Can you work these out from the model? Positions are in its coordinate system, mm. Coordinates: 2 decimals unless noted, no trailing zeros. Order: outer loops, then holes, each group sorted by start corner. A loop starts at its lowest first (then second) coordinate and runs counter-clockwise, first axis right, second up. Notation, with made-up numbers: (5, -22) -> (49, -22) arc R23 cw to (49, 11) -> close; hole circle Ø7 at (45, 5). An arc over 180 degrees is marked (long way). Answer as CSV lines item,"result".
from build123d import *

# Parameters (mm, degrees)
BOSS_EXTRU_1_DEPTH = 10


with BuildPart() as part:
    # Esquisse1 → Boss.-Extru.1 (new body)
    with BuildSketch(Plane(origin=(0, 0, 0), x_dir=(1, 0, 0), z_dir=(0, 1, 0))):
        with BuildLine():
            Line((147.5, -25), (150, -25))
            Line((150, -25), (150, 25))
            Line((150, 25), (-150, 25))
            Line((-150, 25), (-150, -25))
            Line((-150, -25), (-147.5, -25))
            ThreePointArc((-147.5, -25), (-120, 2.5), (-92.5, -25))
            Line((-92.5, -25), (-87.5, -25))
            ThreePointArc((-87.5, -25), (-60, 2.5), (-32.5, -25))
            Line((-32.5, -25), (-27.5, -25))
            ThreePointArc((-27.5, -25), (0, 2.5), (27.5, -25))
            Line((27.5, -25), (32.5, -25))
            ThreePointArc((32.5, -25), (60, 2.5), (87.5, -25))
            Line((87.5, -25), (92.5, -25))
            ThreePointArc((92.5, -25), (120, 2.5), (147.5, -25))
        make_face()
    extrude(amount=BOSS_EXTRU_1_DEPTH)


solid = part.part
Q1. Imagine slicing it at D-D (z = 5). List the corners of the cut face in (x, y) for me.
Solution:
outline,"(-150, 0) -> (-138.87, 0) -> (-138.87, 10) -> (-150, 10) -> close; (-101.13, 0) -> (-78.87, 0) -> (-78.87, 10) -> (-101.13, 10) -> close; (-41.13, 0) -> (-18.87, 0) -> (-18.87, 10) -> (-41.13, 10) -> close; (18.87, 0) -> (41.13, 0) -> (41.13, 10) -> (18.87, 10) -> close; (78.87, 0) -> (101.13, 0) -> (101.13, 10) -> (78.87, 10) -> close; (138.87, 0) -> (150, 0) -> (150, 10) -> (138.87, 10) -> close"
Q2. Imagine slicing it at B-B (y = 1.75). List the corners of the cut face in (x, z) for me, and give its area (3 significant figures).
Solution:
outline,"(-150, -25) -> (150, -25) -> (150, 25) -> (147.5, 25) arc R27.5 cw to (92.5, 25) -> (87.5, 25) arc R27.5 cw to (32.5, 25) -> (27.5, 25) arc R27.5 cw to (-27.5, 25) -> (-32.5, 25) arc R27.5 cw to (-87.5, 25) -> (-92.5, 25) arc R27.5 cw to (-147.5, 25) -> (-150, 25) -> close"
area,"9,060 mm2"
Q3. For P1, Ø4, axis at x = 105, z = -1, coming from the -Y side, with a flat end and sliding along its axis, tell me the tip position at first contact or that it passes through.
Solution:
P1,"y = 0"
Q4. Imagine slicing it at A-A (z = 19.5). List the corners of the cut face in (x, y) for me.
Solution:
outline,"(-150, 0) -> (-146.94, 0) -> (-146.94, 10) -> (-150, 10) -> close; (-93.06, 0) -> (-86.94, 0) -> (-86.94, 10) -> (-93.06, 10) -> close; (-33.06, 0) -> (-26.94, 0) -> (-26.94, 10) -> (-33.06, 10) -> close; (26.94, 0) -> (33.06, 0) -> (33.06, 10) -> (26.94, 10) -> close; (86.94, 0) -> (93.06, 0) -> (93.06, 10) -> (86.94, 10) -> close; (146.94, 0) -> (150, 0) -> (150, 10) -> (146.94, 10) -> close"
Q5. If I drill on line 1 (X direction, y = 1, z = 4); line 2 (X direction, y = 6.25, z = 20); line 3 (Z direction, x = -0.5, y = 1.75), over which ranges is the centre line in solid material (lowest first)?
Solution:
line 1,"-150 to -137.76, -102.24 to -77.76, -42.24 to -17.76, 17.76 to 42.24, 77.76 to 102.24, 137.76 to 150"
line 2,"-150 to -147.04, -92.96 to -87.04, -32.96 to -27.04, 27.04 to 32.96, 87.04 to 92.96, 147.04 to 150"
line 3,"-25 to -2.5"
Q6. Imagine slicing it at C-C (x = 131.5). List the corners of the cut face in (y, z) for me, and give its area (3 significant figures).
Solution:
outline,"(0, -25) -> (10, -25) -> (10, 0.02) -> (0, 0.02) -> close"
area,"250 mm2"
